Check sheet for the modelled part. Datum: model origin and axes. Units: mm. A direction names the side the tool comes from. Round coordinates to 2 decimals unless told otherwise and drop trailing zeros. Write each loop counter-clockwise with the first axis right and the second up, starting at its lowest first coordinate (ties: lowest second). Pieces come first, ordered by that corner, then holes. Notation, with made-up numbers: (65.25, 51.5) -> (89.25, 51.5) arc R34 cw to (89.25, 88.5) -> close; hole circle Ø9 at (88, -37.75). An arc over 180 degrees is marked (long way). One line per item, written item: value.
from build123d import *

# Parameters (mm, degrees)
SKETCH1_R           = 1
BOSS_EXTRUDE1_DEPTH = 2
FILLET1_R           = 2
FILLET2_R           = 1
SKETCH2_R           = 1.5
CUT_EXTRUDE1_DEPTH  = 0.5


with BuildPart() as part:
    # Sketch1 → Boss-Extrude1 (new body)
    with BuildSketch(Plane(origin=(0, 0, 0), x_dir=(1, 0, 0), z_dir=(0, 1, 0))):
        Polygon((1.750249519, 11.413586639), (-10.759580737, -4.191032773), (9.009331218, -7.222553866), align=None)
        with Locations(Location((0.670392162, 5.734449205, 0), (0, 0, 270))):
            Circle(SKETCH1_R, mode=Mode.SUBTRACT)
        with Locations(Location((4.630982607, -3.447801245, 0), (0, 0, 270))):
            Circle(SKETCH1_R, mode=Mode.SUBTRACT)
        with Locations(Location((-5.301374769, -2.28664796, 0), (0, 0, 270))):
            Circle(SKETCH1_R, mode=Mode.SUBTRACT)
    extrude(amount=BOSS_EXTRUDE1_DEPTH)

    # Fillet1
    fillet1_edges = [part.edges().sort_by_distance(p)[0] for p in [
        (9.009331218, 1, 7.222553866),
        (-10.759580737, 1, 4.191032773),
        (1.750249519, 1, -11.413586639),
    ]]
    fillet(fillet1_edges, radius=FILLET1_R)

    # Fillet2
    fillet2_edges = [part.edges().sort_by_distance(p)[0] for p in [
        (-4.504665609, 2, -3.611276933),
        (5.379790368, 2, -2.095516386),
        (-0.875124759, 2, 5.706793319),
        (-8.895966686, 2, 3.465124603),
        (7.448869277, 2, 5.97157084),
        (1.44709741, 2, -9.436695443),
    ]]
    fillet(fillet2_edges, radius=FILLET2_R)

    # Sketch2 → Cut-Extrude1 (cut)
    with BuildSketch(Plane(origin=(0, 2, 0), x_dir=(1, 0, 0), z_dir=(0, 1, 0))):
        with Locations(Location((0.670392162, 5.734449205, 0), (0, 0, 270))):
            Circle(SKETCH2_R)
        with Locations(Location((-5.301374769, -2.28664796, 0), (0, 0, 270))):
            Circle(SKETCH2_R)
        with Locations(Location((4.630982607, -3.447801245, 0), (0, 0, 270))):
            Circle(SKETCH2_R)
    extrude(amount=-CUT_EXTRUDE1_DEPTH, mode=Mode.SUBTRACT)


solid = part.part
Item 1: Depth check by flat-ended pin: P1, Ø0.9, axis at x = 0, z = -6, coming from the +Y side; P2, Ø1, axis at y = 1.5, z = 0.5, coming from the -X side; P3, Ø3, axis at x = -4.5, z = -5, coming from the +Y side. Enter the tip coordinate at first touch or a pass-through.
Answer:
P1: stops at y = 1.5
P2: stops at x = -8.11
P3: stops at y = 1.93
Item 2: Sectioned sample at A-A on y = 0.55. Enter the section's corners in (x, z).
Answer:
outline: (-8.59, 1.49) -> (-0.42, -8.71) arc R2 ccw to (3.01, -8.19) -> (7.75, 3.99) arc R2 ccw to (5.59, 6.7) -> (-7.34, 4.72) arc R2 ccw to start; hole circle Ø2 at (-5.3, 2.29); hole circle Ø2 at (0.67, -5.73); hole circle Ø2 at (4.63, 3.45)
Item 3: Tool access check on faces 1 (the flat face through (-4, 1.5, 2)), 2 (the cylindrical face through (1.42, 0.51, -9.44)). Record the directions out of +Z, -Z, +X, -X, +Y, -Y that give a thin tool (end or side, any length) a straight path to the whole face; none if there is none.
Answer:
face 1: +Y
face 2: -Z, +Y, -Y
Item 4: Thickness scan on line 1 (X direction, y = 1.7, z = 3); line 2 (Z direction, x = -5.25, y = 0.4); line 3 (Z direction, x = 0.75, y = 0.9). Record the ranges inside material, lowest first.
Answer:
line 1: x = -8.73 to -6.62, -3.98 to 3.2, 6.06 to 7.06
line 2: z = -2.68 to 1.29, 3.29 to 5.04
line 3: z = -9.42 to -6.73, -4.74 to 5.96
Item 5: Mould release check, pull along Z, two halves, no side actions. Record for faces 3 (the flat face through (5.413, 0.493, -2.01)), 4 (the cylindrical face through (-0.74, 1.7, 5.44)), 5 (the cylindrical face through (-4.29, 1.75, 1.18)): pulls with the +Z half, pulls with the -Z half, needs draft (parallel to the pull), parting line crosses it, or undercut.
Answer:
face 3: pulls with the -Z half
face 4: pulls with the +Z half
face 5: undercut
